Design review of the part built by this model. Coordinates are the model's own, in mm. A direction names the side the tool comes from. Give positions to 0.01 mm unless a question says otherwise; leave off trailing zeros. Write each loop counter-clockwise with the first axis right and the second up, starting at its lowest first coordinate (ties: lowest second). Pieces come first, ordered by that corner, then holes. Notation, with made-up numbers: M 66,78.25 L 87,78.25 A17 ccw 87,84.25 Z; hole C 12,-21.5 d7. An arc over 180 degrees is marked long. Answer in a Markdown table with one row per item.
```python
from build123d import *

# Parameters (mm, degrees)
F0_W     = 25
F0_H     = 2
F1_DEPTH = 25
F2_R     = 1
F3_DEPTH = 25
F4_DEPTH = 5
F6_DEPTH = 20


with BuildPart() as f1:
    # F0 (on Front) → F1 (new body)
    with BuildSketch(Plane.XZ):
        with Locations((-1.9524786621, -32.3955392072)):
            Rectangle(F0_W, F0_H)
    extrude(amount=F1_DEPTH)

    # F2 (on face) → F3 (cut)
    with BuildSketch(Plane.XY.offset(-31.3955392072)):
        with Locations((-1.9404253719, -20.35)):
            Circle(F2_R)
        with Locations((5.8975151656, -6.7464457538)):
            Circle(F2_R)
        with Locations((-9.8024786621, -6.760367258)):
            Circle(F2_R)
    extrude(amount=-F3_DEPTH, mode=Mode.SUBTRACT)

    # F4 (add): a face of the model
    f4_faces = [f1.faces().sort_by_distance(p)[0] for p in [
        (-1.9524786621, 0, -32.3955392072),
    ]]
    extrude(f4_faces, amount=F4_DEPTH)

    # F5 (on face) → F6 (join)
    with BuildSketch(Plane.XY.offset(-31.3955392072)):
        Polygon((-14.4524786621, 5), (-14.4524786621, 3), (10.433112914, 3), (10.5475213379, 3), (10.5475213379, 5), align=None)
    extrude(amount=F6_DEPTH)


solid = f1.part
```
1) To check wall thickness, follow probe 1 along Z at (x, y) = (2, -13.25); probe 2 along Y at (x, z) = (-12.5, -13.5). State the ranges of each line that lie inside material, in increasing order. Write a range as [from, to].
Geometry says:
| item | result |
|---|---|
| probe 1 | [-33.4, -31.4] |
| probe 2 | [3, 5] |
2) Add section B-B (x = 6). Write out the cut boundary in (y, z).
Geometry says:
| item | result |
|---|---|
| outline | M -25,-33.4 L -7.74,-33.4 L -7.74,-31.4 L -25,-31.4 Z; M -5.75,-33.4 L 5,-33.4 L 5,-11.4 L 3,-11.4 L 3,-31.4 L -5.75,-31.4 Z |
3) Add section C-C (x = 0.75). Write out the cut boundary in (y, z), and give its area (3 significant figures).
Geometry says:
| item | result |
|---|---|
| outline | M -25,-33.4 L 5,-33.4 L 5,-11.4 L 3,-11.4 L 3,-31.4 L -25,-31.4 Z |
| area | 100 mm^2 |
4) For faces 5 (the face through (-2, -11, -31.396)), 6 (the face through (-2, -25, -32)), list the 3-axis set-ups (+Z, -Z, +X, -X, +Y, -Y) from which the entire face can be reached by the end or side of a thin tool; tool diameter is ignored.
Geometry says:
| item | result |
|---|---|
| face 5 | +Z, +X, -X, -Y |
| face 6 | +Z, -Z, +X, -X, -Y |
5) The part is to be moulded in two halves that separate along X. For faces 1 (the face through (10.548, -3, -32)), 2 (the face through (-14.452, -4, -32)), 3 (the face through (-2, 5, -23)), 4 (the face through (5.16, -6.07, -32.38)), say which applies: released by +X, released by -X, zero draft, split by the parting line, or undercut.
Geometry says:
| item | result |
|---|---|
| face 1 | released by +X |
| face 2 | released by -X |
| face 3 | zero draft |
| face 4 | undercut |
6) Add section D-D (z = -15.75). Write out the cut boundary in (x, y), and give its area (3 significant figures).
Geometry says:
| item | result |
|---|---|
| outline | M -14.45,3 L 10.55,3 L 10.55,5 L -14.45,5 Z |
| area | 50.0 mm^2 |
7) Add section A-A (y = -20.35). Write out the cut boundary in (x, z).
Geometry says:
| item | result |
|---|---|
| outline | M -14.45,-33.4 L -2.94,-33.4 L -2.94,-31.4 L -14.45,-31.4 Z; M -0.94,-33.4 L 10.55,-33.4 L 10.55,-31.4 L -0.94,-31.4 Z |
8) Insertion check: P1, Ø2, axis at x = -0.5, z = -15, coming from the -Y side; P2, Ø3, axis at y = -18.5, z = -29.5, coming from the +X side; P3, Ø1, axis at x = -11, y = -12.5, coming from the +Z side. Each pin has a flat end and moves straight along its axis. Give the tip position at first contact, or say it passes through.
Geometry says:
| item | result |
|---|---|
| P1 | y = 3 |
| P2 | through |
| P3 | z = -31.4 |
